Can you work these out from the model? Positions are in its coordinate system, mm. Face numbers are marked on the shaded views. Give positions to 0.01 mm unless a question says otherwise; leave off trailing zeros. Write each loop counter-clockwise with the first axis right and the second up, starting at its lowest first coordinate (ties: lowest second). Pieces come first, ordered by that corner, then holes. Notation, with made-up numbers: M 1,85 L 23,85 A20 ccw 23,120 Z; hole C 85.25,75.5 d2. An arc over 180 degrees is marked long. Write each question's results on one line, items separated by ' | '.
from build123d import *

# Parameters (mm, degrees)
CUT_EXTRUDE1_DEPTH      = 6.830951895
CUT_EXTRUDE1_DEPTH_BACK = 6.830951895
CUT_EXTRUDE2_DEPTH      = 6.830951895
CUT_EXTRUDE2_DEPTH_BACK = 6.830951895
SKETCH3_W               = 8
SKETCH3_H               = 0.5
SKETCH3_W_2             = 4.333333333


with BuildPart() as part:
    # Sketch1 → Revolve1 (revolve)
    with BuildSketch(Plane.XY, mode=Mode.PRIVATE) as revolve1_sk:
        Polygon((0, 0), (0, 1.6), (4, 1.6), (4, 3), (-4, 3), (-4, 0), align=None)
    revolve(revolve1_sk.sketch.rotate(Axis((0, 0, 0), (1, 0, 0)), 90), axis=Axis((0, 0, 0), (1, 0, 0)))

    # Sketch2 → Cut-Extrude1 (cut, two sides: drawn at the far end of the back side and taken through both)
    with BuildSketch(Plane(origin=(0, 0, 0), x_dir=(1, 0, 0), z_dir=(0, 1, 0)).offset(-CUT_EXTRUDE1_DEPTH_BACK)):
        Polygon((-4, -3), (0, 3), (-4, 3), align=None)
    extrude(amount=CUT_EXTRUDE1_DEPTH + CUT_EXTRUDE1_DEPTH_BACK, mode=Mode.SUBTRACT)

    # Sketch3 → Cut-Extrude2 (cut, two sides: drawn at the far end of the back side and taken through both)
    with BuildSketch(Plane(origin=(0, 0, 0), x_dir=(1, 0, 0), z_dir=(0, 1, 0)).offset(-CUT_EXTRUDE2_DEPTH_BACK)):
        with Locations((0, -2.75)):
            Rectangle(SKETCH3_W, SKETCH3_H)
        with Locations((1.833333333, 2.75)):
            Rectangle(SKETCH3_W_2, SKETCH3_H)
    extrude(amount=CUT_EXTRUDE2_DEPTH + CUT_EXTRUDE2_DEPTH_BACK, mode=Mode.SUBTRACT)


solid = part.part
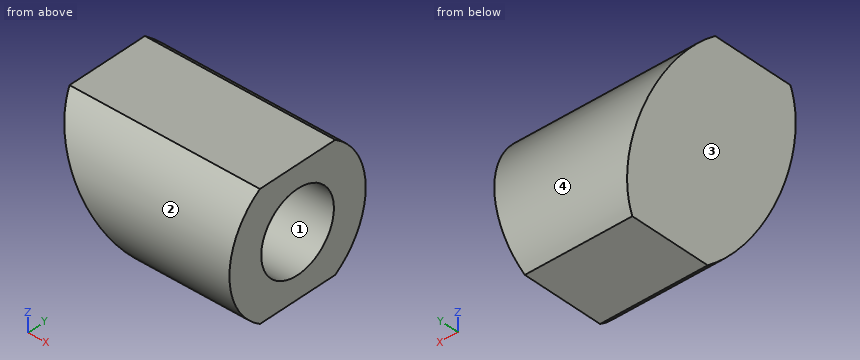
Item 1: I'm going to push flat-ended pins straight in: pin 1 (2 mm diameter, centred on y = -2, z = -1, fed in from -X); pin 2 (2 mm diameter, centred on x = -1.5, z = 1.5, fed in from +Y). Where does each tip first touch, or does it pass through?
Geometry says:
pin 1: stops at x = -2 | pin 2: stops at y = 2.96
Item 2: If I drill on line 1 (Y direction, x = 2.9, z = 0); line 2 (Y direction, x = 3, z = -0.8); line 3 (Z direction, x = 2.25, y = 1.3), over which ranges is the centre line in solid material (lowest first)? Write a range as from..to.
Geometry says:
line 1: y = -3..-1.6, 1.6..3 | line 2: y = -2.89..-1.39, 1.39..2.89 | line 3: z = -2.5..-0.93, 0.93..2.5
Item 3: I want a section at D-D, the plane x = -1. Please give me the cut outline in (y, z).
Geometry says:
outline: M -2.6,-1.5 L 2.6,-1.5 A3 ccw 1.66,2.5 L -1.66,2.5 A3 ccw Z
Item 4: Thinking about a two-plate mould opening in Y: for the marked faces 1, 2, 3 and 4, which applies, +Y half, -Y half, draft (parallel to the pull), parting line (faces both ways), or undercut?
Geometry says:
face 1: undercut | face 2: -Y half | face 3: draft | face 4: +Y half
Item 5: I want a section at C-C, the plane z = 0. Please give me the cut outline in (x, y), and give its area (3 significant figures).
Geometry says:
outline: M -2,-3 L 4,-3 L 4,-1.6 L 0,-1.6 L 0,1.6 L 4,1.6 L 4,3 L -2,3 Z | area: 23.2 mm2
Item 6: I want a section at A-A, the plane x = 3.25. Please give me the cut outline in (y, z).
Geometry says:
outline: M -1.66,-2.5 L 1.66,-2.5 A3 ccw 1.66,2.5 L -1.66,2.5 A3 ccw Z; hole C 0,0 d3.2
Item 7: I want a section at B-B, the plane y = 0. Please give me the cut outline in (x, z).
Geometry says:
outline: M -3.67,2.5 L -0.33,-2.5 L 4,-2.5 L 4,-1.6 L 0,-1.6 L 0,1.6 L 4,1.6 L 4,2.5 Z
